Here's how the part is built. I have some questions about the finished solid (model axes, mm). A direction names the side the tool comes from. Give positions to 0.01 mm unless a question says otherwise; leave off trailing zeros. Loops run counter-clockwise (first coordinate to the right, second up) from the corner with the lowest first, then second, coordinate; pieces in that order, holes last. Notation, with made-up numbers: (64.5, 69.25) - (75.5, 69.25) arc R16 cw to (75.5, 77.25) - close; hole circle Ø11 at (46, 12.5). An arc over 180 degrees is marked (long way). Use one line per item in the form item = value.
from build123d import *

# Parameters (mm, degrees)
F0_W     = 32
F0_H     = 32
F1_DEPTH = 32
F2_W     = 32
F2_H     = 32
F3_DEPTH = 18
F4_W     = 32
F4_H     = 32
F5_DEPTH = 18
F6_W     = 28.5
F6_H     = 28.5
F7_DEPTH = 35
F8_W     = 28.5
F8_H     = 28.5
F9_DEPTH = 35


with BuildPart() as f1:
    # F0 (on Front) → F1 (new body)
    with BuildSketch(Plane.XZ):
        Rectangle(F0_W, F0_H)
    extrude(amount=F1_DEPTH)

    # F2 (on face) → F3 (join)
    with BuildSketch(Plane.XY.offset(16)):
        with Locations((0, -16)):
            Rectangle(F2_W, F2_H)
    extrude(amount=F3_DEPTH)

    # F4 (on face) → F5 (join)
    with BuildSketch(Plane.XZ.offset(32)):
        Rectangle(F4_W, F4_H)
    extrude(amount=F5_DEPTH)

    # F6 (on face) → F7 (join)
    with BuildSketch(Plane.XY.offset(34)):
        with Locations((0, -16)):
            Rectangle(F6_W, F6_H)
    extrude(amount=F7_DEPTH)

    # F8 (on face) → F9 (join)
    with BuildSketch(Plane.XZ.offset(50)):
        Rectangle(F8_W, F8_H)
    extrude(amount=F9_DEPTH)


solid = f1.part
(1) For faces 1 (the flat face through (0, -32, 25)), 2 (the flat face through (0, -1.75, 51)), 3 (the flat face through (14.25, -67, 0)), which set-ups out of +Z, -Z, +X, -X, +Y, -Y let a thin tool reach every point of the face, with its end or its side?
Geometry says:
face_1 = +Z, +X, -X, -Y
face_2 = +Z, +X, -X, +Y
face_3 = +Z, -Z, +X, -Y
(2) If we section it at C-C (y = -13): List the corners of the cut face in (x, z) for me.
Geometry says:
outline = (-16, -16) - (16, -16) - (16, 34) - (14.25, 34) - (14.25, 69) - (-14.25, 69) - (-14.25, 34) - (-16, 34) - close
(3) If we section it at B-B (x = 5): List the corners of the cut face in (y, z) for me.
Geometry says:
outline = (-85, -14.25) - (-50, -14.25) - (-50, -16) - (0, -16) - (0, 34) - (-1.75, 34) - (-1.75, 69) - (-30.25, 69) - (-30.25, 34) - (-32, 34) - (-32, 16) - (-50, 16) - (-50, 14.25) - (-85, 14.25) - close
(4) For P1, Ø14, axis at x = -3, z = 58.5, coming from the +Y side; P2, Ø8.5, axis at y = -16, z = 52, coming from the -X side; P3, Ø4, axis at y = -26, z = 47.5, coming from the +X side, each with a flat end and sliding along its axis, tell me the tip position at first contact or that it passes through.
Geometry says:
P1 = -1.75
P2 = -14.25
P3 = 14.25
(5) If I drill on probe 1 along Y at (x, z) = (-6.5, 48); probe 2 along X at (y, z) = (-68.5, 6.5); probe 3 along Z at (x, y) = (-10, -48), over which ranges is the centre line in solid material (lowest first)?
Geometry says:
probe_1 = -30.25 to -1.75
probe_2 = -14.25 to 14.25
probe_3 = -16 to 16
(6) If we section it at A-A (z = 8.5): List the corners of the cut face in (x, y) for me.
Geometry says:
outline = (-16, -50) - (-14.25, -50) - (-14.25, -85) - (14.25, -85) - (14.25, -50) - (16, -50) - (16, 0) - (-16, 0) - close
(7) If we section it at D-D (y = -55): List the corners of the cut face in (x, z) for me, plus the area to 3 significant figures.
Geometry says:
outline = (-14.25, -14.25) - (14.25, -14.25) - (14.25, 14.25) - (-14.25, 14.25) - close
area = 812 mm²
